Verification items for the finished model (mm, model axes). Face numbers are marked on the shaded views. A direction names the side the tool comes from. Round coordinates to 2 decimals unless told otherwise and drop trailing zeros. Loops run counter-clockwise (first coordinate to the right, second up) from the corner with the lowest first, then second, coordinate; pieces in that order, holes last.
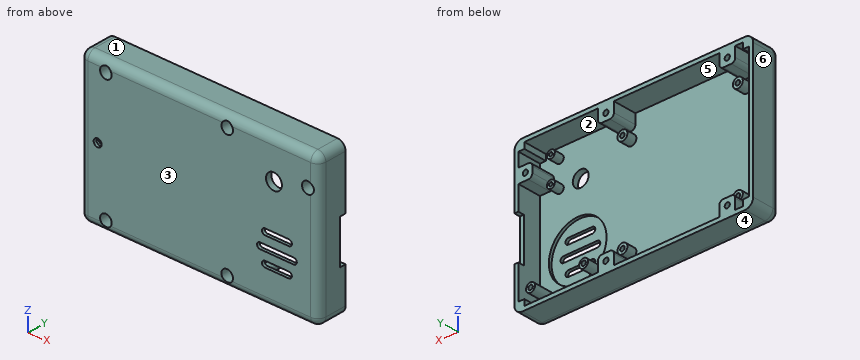
from build123d import *

# Parameters (mm, degrees)
SKETCH1_W                   = 120
SKETCH1_H                   = 75
MAIN_STRUCTURE_DEPTH        = 15
SKETCH2_W                   = 116
SKETCH2_H                   = 71
INSIDE_CUT_DEPTH            = 12
SKETCH3_R                   = 2.5
SKETCH3_R_2                 = 1.15
PI_STANDOFFS_DEPTH          = 5
SKETCH4_R                   = 2
SKETCH4_R_2                 = 0.9
CAMERA_STANDOFFS_DEPTH      = 5
BODY_FILLET_1_R             = 4
BODY_FILLET_2_R             = 4
BODY_FILLET_3_R             = 4
BODY_FILLET_4_R             = 4
SKETCH5_R                   = 2.25
SKETCH5_R_2                 = 1.15
FONA_STANDOFFS_DEPTH        = 13
SKETCH6_W                   = 3
SKETCH6_H                   = 3
CORNER_SUPPORT_DEPTH        = 12
SKETCH8_W                   = 22
SKETCH8_H                   = 3
CHARGER_CUTOUT_DEPTH        = 10
SKETCH9_W                   = 8
SKETCH9_H                   = 7
SKETCH9_W_2                 = 7
MOUNTING_STRUCTURE_DEPTH    = 12
MOUNTING_STRUCTURE_FILLET_R = 2
SKETCH10_R                  = 1.3
CASE_MOUNTING_HOLES_DEPTH   = 15
SKETCH13_R                  = 2.9
CASE_SCREW_HEAD_HOLES_DEPTH = 8.85
SKETCH14_R                  = 14.5
SPEAKER_HOLDER_DEPTH        = 1.5
SOUND_CUTOUT_DEPTH          = 1.5
SKETCH25_R                  = 2.5
MICROPHONE_HOLDER_DEPTH     = 1.5
SKETCH26_R                  = 2
MICROPHONE_CUTOUT_DEPTH     = 1.5
SKETCH27_R                  = 4
CAMERA_CUTOUT_DEPTH         = 10


with BuildPart() as part:
    # Sketch1 → Main Structure (new body)
    with BuildSketch(Plane(origin=(0, 0, 0), x_dir=(1, 0, 0), z_dir=(0, 1, 0))):
        Rectangle(SKETCH1_W, SKETCH1_H)
    extrude(amount=MAIN_STRUCTURE_DEPTH)

    # Sketch2 → Inside Cut (cut)
    with BuildSketch(Plane(origin=(0, 15, 0), x_dir=(1, 0, 0), z_dir=(0, 1, 0))):
        Rectangle(SKETCH2_W, SKETCH2_H)
    extrude(amount=-INSIDE_CUT_DEPTH, mode=Mode.SUBTRACT)

    # Sketch3 → Pi Standoffs (add)
    with BuildSketch(Plane(origin=(0, 3, 0), x_dir=(1, 0, 0), z_dir=(0, 1, 0))):
        with Locations((-46, -24.5)):
            Circle(SKETCH3_R)
        with Locations((-46, -24.5)):
            Circle(SKETCH3_R_2, mode=Mode.SUBTRACT)
        with Locations((-46, 24.5)):
            Circle(SKETCH3_R)
        with Locations((-46, 24.5)):
            Circle(SKETCH3_R_2, mode=Mode.SUBTRACT)
        with Locations((12, 24.5)):
            Circle(SKETCH3_R)
        with Locations((12, 24.5)):
            Circle(SKETCH3_R_2, mode=Mode.SUBTRACT)
        with Locations((12, -24.5)):
            Circle(SKETCH3_R)
        with Locations((12, -24.5)):
            Circle(SKETCH3_R_2, mode=Mode.SUBTRACT)
    extrude(amount=PI_STANDOFFS_DEPTH)

    # Sketch4 → Camera Standoffs (add)
    with BuildSketch(Plane(origin=(0, 3, 0), x_dir=(1, 0, 0), z_dir=(0, 1, 0))):
        with Locations((48, -30.5)):
            Circle(SKETCH4_R)
        with Locations((48, -30.5)):
            Circle(SKETCH4_R_2, mode=Mode.SUBTRACT)
        with Locations((48, -17.5)):
            Circle(SKETCH4_R)
        with Locations((48, -17.5)):
            Circle(SKETCH4_R_2, mode=Mode.SUBTRACT)
    extrude(amount=CAMERA_STANDOFFS_DEPTH)

    # Body Fillet 1
    body_fillet_1_edges = [part.edges().sort_by_distance(p)[0] for p in [
        (-60, 0, 0),
    ]]
    fillet(body_fillet_1_edges, radius=BODY_FILLET_1_R)

    # Body Fillet 2
    body_fillet_2_edges = [part.edges().sort_by_distance(p)[0] for p in [
        (2, 0, -37.5),
        (-58.828427125, 1.171572875, -37.5),
        (-60, 9.5, -37.5),
    ]]
    fillet(body_fillet_2_edges, radius=BODY_FILLET_2_R)

    # Body Fillet 3
    body_fillet_3_edges = [part.edges().sort_by_distance(p)[0] for p in [
        (2, 0, 37.5),
        (-58.828427125, 1.171572875, 37.5),
        (-60, 9.5, 37.5),
    ]]
    fillet(body_fillet_3_edges, radius=BODY_FILLET_3_R)

    # Body Fillet 4
    body_fillet_4_edges = [part.edges().sort_by_distance(p)[0] for p in [
        (60, 9.5, 37.5),
        (60, 9.5, -37.5),
        (60, 1.171572875, -36.328427125),
        (60, 0, 0),
        (60, 1.171572875, 36.328427125),
    ]]
    fillet(body_fillet_4_edges, radius=BODY_FILLET_4_R)

    # Sketch5 → Fona Standoffs (add)
    with BuildSketch(Plane(origin=(0, 3, 0), x_dir=(1, 0, 0), z_dir=(0, 1, 0))):
        with Locations((24.33, 29.5)):
            Circle(SKETCH5_R)
        with Locations((24.33, 29.5)):
            Circle(SKETCH5_R_2, mode=Mode.SUBTRACT)
        with Locations((51, 29.5)):
            Circle(SKETCH5_R)
        with Locations((51, 29.5)):
            Circle(SKETCH5_R_2, mode=Mode.SUBTRACT)
    extrude(amount=FONA_STANDOFFS_DEPTH)

    # Sketch6 → Corner Support (add)
    with BuildSketch(Plane(origin=(0, 3, 0), x_dir=(1, 0, 0), z_dir=(0, 1, 0))):
        with Locations((-56.5, -34)):
            Rectangle(SKETCH6_W, SKETCH6_H)
        with Locations((-56.5, 34)):
            Rectangle(SKETCH6_W, SKETCH6_H)
        with Locations((56.5, -34)):
            Rectangle(SKETCH6_W, SKETCH6_H)
        with Locations((56.5, 34)):
            Rectangle(SKETCH6_W, SKETCH6_H)
    extrude(amount=CORNER_SUPPORT_DEPTH)

    # Sketch8 → Charger Cutout (cut)
    with BuildSketch(Plane(origin=(60, 0, 0), x_dir=(0, 0, -1), z_dir=(1, 0, 0))):
        with Locations((4.5, 13.5)):
            Rectangle(SKETCH8_W, SKETCH8_H)
    extrude(amount=-CHARGER_CUTOUT_DEPTH, mode=Mode.SUBTRACT)

    # Sketch9 → Mounting Structure (add)
    with BuildSketch(Plane(origin=(0, 3, 0), x_dir=(1, 0, 0), z_dir=(0, 1, 0))):
        with Locations((-47, -32)):
            Rectangle(SKETCH9_W, SKETCH9_H)
        with Locations((54.5, -22)):
            Rectangle(SKETCH9_W_2, SKETCH9_H)
        with Locations((-47, 32)):
            Rectangle(SKETCH9_W, SKETCH9_H)
        with Locations((14, 32)):
            Rectangle(SKETCH9_W, SKETCH9_H)
        with Locations((14, -32)):
            Rectangle(SKETCH9_W, SKETCH9_H)
    extrude(amount=MOUNTING_STRUCTURE_DEPTH)

    # Mounting Structure Fillet
    mounting_structure_fillet_edges = [part.edges().sort_by_distance(p)[0] for p in [
        (-43, 9, 28.5),
        (-51, 9, 28.5),
        (51, 9, 18.5),
        (51, 9, 25.5),
        (-43, 9, -28.5),
        (-51, 9, -28.5),
        (18, 9, -28.5),
        (10, 9, -28.5),
        (18, 9, 28.5),
        (10, 9, 28.5),
    ]]
    fillet(mounting_structure_fillet_edges, radius=MOUNTING_STRUCTURE_FILLET_R)

    # Sketch10 → Case Mounting Holes (cut)
    with BuildSketch(Plane(origin=(0, 15, 0), x_dir=(1, 0, 0), z_dir=(0, 1, 0))):
        with Locations((-47, 32)):
            Circle(SKETCH10_R)
        with Locations((-47, -32)):
            Circle(SKETCH10_R)
        with Locations((14, -32)):
            Circle(SKETCH10_R)
        with Locations((14, 32)):
            Circle(SKETCH10_R)
        with Locations((54.5, -22)):
            Circle(SKETCH10_R)
    extrude(amount=-CASE_MOUNTING_HOLES_DEPTH, mode=Mode.SUBTRACT)

    # Sketch13 → Case Screw Head Holes (cut)
    with BuildSketch(Plane.XZ):
        with Locations((-47, 32)):
            Circle(SKETCH13_R)
        with Locations((14, 32)):
            Circle(SKETCH13_R)
        with Locations((14, -32)):
            Circle(SKETCH13_R)
        with Locations((-47, -32)):
            Circle(SKETCH13_R)
        with Locations((54.5, 22)):
            Circle(SKETCH13_R)
    extrude(amount=-CASE_SCREW_HEAD_HOLES_DEPTH, mode=Mode.SUBTRACT)

    # Sketch14 → Speaker Holder (cut)
    with BuildSketch(Plane(origin=(0, 3, 0), x_dir=(1, 0, 0), z_dir=(0, 1, 0))):
        with Locations((39, 12.5)):
            Circle(SKETCH14_R)
    extrude(amount=-SPEAKER_HOLDER_DEPTH, mode=Mode.SUBTRACT)

    # Sketch23 → Sound Cutout (cut)
    with BuildSketch(Plane(origin=(0, 1.5, 0), x_dir=(1, 0, 0), z_dir=(0, 1, 0))):
        with BuildLine():
            Line((33, 21), (45, 21))
            ThreePointArc((45, 21), (46.5, 19.5), (45, 18))
            Line((45, 18), (33, 18))
            ThreePointArc((33, 18), (31.5, 19.5), (33, 21))
        make_face()
        with BuildLine():
            Line((30.5, 14), (47.5, 14))
            ThreePointArc((47.5, 14), (49, 12.5), (47.5, 11))
            Line((47.5, 11), (30.5, 11))
            ThreePointArc((30.5, 11), (29, 12.5), (30.5, 14))
        make_face()
        with BuildLine():
            Line((33, 7), (45, 7))
            ThreePointArc((45, 7), (46.5, 5.5), (45, 4))
            Line((45, 4), (33, 4))
            ThreePointArc((33, 4), (31.5, 5.5), (33, 7))
        make_face()
    extrude(amount=-SOUND_CUTOUT_DEPTH, mode=Mode.SUBTRACT)

    # Sketch25 → Microphone holder (cut)
    with BuildSketch(Plane(origin=(0, 3, 0), x_dir=(1, 0, 0), z_dir=(0, 1, 0))):
        with Locations((-51.147743093, 0)):
            Circle(SKETCH25_R)
    extrude(amount=-MICROPHONE_HOLDER_DEPTH, mode=Mode.SUBTRACT)

    # Sketch26 → Microphone Cutout (cut)
    with BuildSketch(Plane(origin=(0, 1.5, 0), x_dir=(1, 0, 0), z_dir=(0, 1, 0))):
        with Locations((-51.147743093, 0)):
            Circle(SKETCH26_R)
    extrude(amount=-MICROPHONE_CUTOUT_DEPTH, mode=Mode.SUBTRACT)

    # Sketch27 → Camera Cutout (cut)
    with BuildSketch(Plane(origin=(0, 3, 0), x_dir=(1, 0, 0), z_dir=(0, 1, 0))):
        with Locations((37.5, -18)):
            Circle(SKETCH27_R)
    extrude(amount=-CAMERA_CUTOUT_DEPTH, mode=Mode.SUBTRACT)


solid = part.part
1. Section check C-C (z = 12). Enter the section's corners in (x, y).
2. Tool access check on the marked faces 5 and 6. Record the directions out of +Z, -Z, +X, -X, +Y, -Y that give a thin tool (end or side, any length) a straight path to the whole face; none if there is none.
3. Scan lines: L1, parallel to X at y = 11.5, z = 22; L2, parallel to X at y = 12.25, z = -32; L3, parallel to X at y = 8.5, z = 17.5. Record each from-to range of solid material in increasing order.
4. Gauge pin test, flat ends, axial feed: P1, Ø1.1, axis at x = 48, z = 30.5, coming from the +Y side; P2, Ø0.8, axis at x = 36, y = 1, coming from the +Z side; P3, Ø1.4, axis at x = 48.5, z = 17.5, coming from the +Y side. Record the tip position at first contact, or that the pin passes through.
5. Release check for a two-part mould opening along Z. For the marked faces 1, 2, 3 and 4 record: released by +Z, released by -Z, zero draft, split by the parting line, or undercut.
6. Section check B-B (y = 10.75). Give the number of separate pieces and of enclosed holes in the cut face, then the cut area to 3 significant figures.
7. Section check A-A (z = -12.5). Enter the section's corners in (x, y), then the cut area to 3 significant figures.
Taken from the geometry:
1. outline: (-60, 4) arc R4 ccw to (-56, 0) - (56, 0) arc R4 ccw to (60, 4) - (60, 15) - (58, 15) - (58, 3) - (-58, 3) - (-58, 15) - (-60, 15) - close
2. face 5: +Y
2. face 6: +Z, -Z, -X, +Y, -Y
3. L1: x = -60 to -58, 51 to 53.2, 55.8 to 60
3. L2: x = -60 to -58, -51 to -48.3, -45.7 to -43, 10 to 12.7, 15.3 to 18, 58 to 60
3. L3: x = -60 to -58, 58 to 60
4. P1: stops at y = 3
4. P2: stops at z = 36.54
4. P3: stops at y = 8
5. face 1: released by +Z
5. face 2: undercut
5. face 3: zero draft
5. face 4: released by -Z
6. separate pieces: 3
6. enclosed holes: 8
6. area: 1,050 mm2
7. outline: (-60, 4) arc R4 ccw to (-56, 0) - (29, 0) - (29, 1.5) - (24.5, 1.5) - (24.5, 3) - (-58, 3) - (-58, 15) - (-60, 15) - close; (49, 0) - (56, 0) arc R4 ccw to (60, 4) - (60, 12) - (58, 12) - (58, 3) - (53.5, 3) - (53.5, 1.5) - (49, 1.5) - close
7. area: 322 mm2
